from build123d import *

# Parameters (mm, degrees)
F1_DEPTH       = 15
F3_D           = 4.5
F3_CSINK_D     = 9
F3_CSINK_ANGLE = 90
F4_R           = 4
F5_R           = 1.5
F6_W           = 3
F6_H           = 8
F7_DEPTH       = 0.5
F8_R           = 1


with BuildPart() as f1:
    # F0 (on Right) → F1 (new body, symmetric)
    with BuildSketch(Plane.YZ):
        Polygon((0, 4.5), (0, 0), (9, 0), (9, 7.5), (-11, 7.5), (-11, 4.5), align=None)
    extrude(amount=F1_DEPTH, both=True)

    # F3 (through all)
    with Locations(Plane.XY.offset(7.5)):
        with Locations((-9, 3.5), (9, 3.5)):
            CounterSinkHole(F3_D / 2, F3_CSINK_D / 2, counter_sink_angle=F3_CSINK_ANGLE)

    # F4
    f4_edges = [f1.edges().sort_by_distance(p)[0] for p in [
        (15, -11, 6),
        (-15, -11, 6),
        (15, 0, 2.25),
        (-15, 0, 2.25),
        (-15, 9, 3.75),
        (15, 9, 3.75),
    ]]
    fillet(f4_edges, radius=F4_R)

    # F5
    f5_edges = [f1.edges().sort_by_distance(p)[0] for p in [
        (-15, -3.5, 4.5),
    ]]
    fillet(f5_edges, radius=F5_R)

    # F6 (on face) → F7 (cut)
    with BuildSketch(Plane.XY.offset(7.5)):
        with Locations((0, 3.5)):
            Rectangle(F6_W, F6_H)
    extrude(amount=-F7_DEPTH, mode=Mode.SUBTRACT)

    # F8
    f8_edges = [f1.edges().sort_by_distance(p)[0] for p in [
        (-1.5, 7.5, 7.25),
        (-1.5, -0.5, 7.25),
        (1.5, -0.5, 7.25),
        (1.5, 7.5, 7.25),
    ]]
    fillet(f8_edges, radius=F8_R)


solid = f1.part
Geometry: final body of the model. Coordinates: model frame, mm. A direction names the side the tool comes from. Coordinates: 2 decimals unless noted, no trailing zeros. Loops run counter-clockwise (first coordinate to the right, second up) from the corner with the lowest first, then second, coordinate; pieces in that order, holes last. Notation, with made-up numbers: (26, 68) - (82, 68) arc R19 ccw to (82, 77) - close; hole circle Ø1 at (26.5, -39). An arc over 180 degrees is marked (long way). One line per question, with ' | ' between items. Start each with the question number.
(1) Cut plane C-C on z = 2. Output: boundary loops of the cut face in (x, y).
(2) Draft query along X for faces 6 (the cylindrical face through (-0.15, -10.55, 4.93)), 7 (the cylindrical face through (14.55, -2.8, 4.93)), 8 (the flat face through (-15, 0.3, 6.3)), 9 (the cylindrical face through (10.786, 2.131, 2.588)). Return one class per face: +X half, -X half, draft (parallel to the pull), parting line (faces both ways), or undercut.
(3) Cut plane B-B on y = 3.5. Output: boundary loops of the cut face in (x, z).
(4) Reachability of faces 1 (the cylindrical face through (-13.797, 7.859, 3.802)), 2 (the cylindrical face through (-1.199, -0.215, 7.246)), 3 (the cylindrical face through (-14.55, -2.65, 4.93)), 4 (the cylindrical face through (13.797, 1.141, 2.291)), 5 (the cylindrical face through (13.797, 7.859, 3.802)) from +Z, -Z, +X, -X, +Y, -Y: full face, straight path, thin tool, end or side. Return the list, or none.
(5) First-contact query: pin 1 (1.5 mm diameter, centred on y = -8, z = 2, fed in from +X); pin 2 (1 mm diameter, centred on x = 5.5, z = 2, fed in from -Y); pin 3 (2 mm diameter, centred on x = 11.5, z = 2.5, fed in from +Y); pin 4 (8.5 mm diameter, centred on x = 4.5, y = -6, fed in from -Z). Flat tips, straight axial feed; report the tip coordinate or a pass-through.
(6) Cut plane D-D on y = -4.5. Output: boundary loops of the cut face in (x, z).
(7) Ray query, L1, parallel to X at y = 3.5, z = 2.15; L2, parallel to Y at x = -9, z = 1.4; L3, parallel to Z at x = -4.5, y = -7.25. Return the intervals inside material, ascending. Write a range as from..to.
(8) Cut plane A-A on x = -9. Output: boundary loops of the cut face in (y, z).
Here are the results:
1) outline: (-15, 4) arc R4 ccw to (-11, 0) - (11, 0) arc R4 ccw to (15, 4) - (15, 5) arc R4 ccw to (11, 9) - (-11, 9) arc R4 ccw to (-15, 5) - close; hole circle Ø4.5 at (-9, 3.5); hole circle Ø4.5 at (9, 3.5)
2) face 6: draft | face 7: +X half | face 8: -X half | face 9: undercut
3) outline: (-15, 6) arc R1.5 ccw to (-14.97, 5.69) - (-14.97, 0) - (-11.25, 0) - (-11.25, 5.25) - (-13.5, 7.5) - (-15, 7.5) - close; (-6.75, 0) - (6.75, 0) - (6.75, 5.25) - (4.5, 7.5) - (1.5, 7.5) - (1.5, 7) - (-1.5, 7) - (-1.5, 7.5) - (-4.5, 7.5) - (-6.75, 5.25) - close; (11.25, 0) - (14.97, 0) - (14.97, 5.69) arc R1.5 ccw to (15, 6) - (15, 7.5) - (13.5, 7.5) - (11.25, 5.25) - close
4) face 1: +Z, -Z, -X, +Y | face 2: +Z | face 3: -Z, -X, -Y | face 4: -Z, +X, -Y | face 5: +Z, -Z, +X, +Y
5) pin 1: through | pin 2: y = 0 | pin 3: y = 9 | pin 4: z = 4.5
6) outline: (-15, 6) arc R1.5 ccw to (-13.5, 4.5) - (13.5, 4.5) arc R1.5 ccw to (15, 6) - (15, 7.5) - (-15, 7.5) - close
7) L1: -14.97..-11.25, -6.75..6.75, 11.25..14.97 | L2: 0..1.25, 5.75..9 | L3: 4.5..7.5
8) outline: (-11, 6) arc R1.5 ccw to (-9.5, 4.5) - (0, 4.5) - (0, 0) - (1.25, 0) - (1.25, 5.25) - (-1, 7.5) - (-11, 7.5) - close; (5.75, 0) - (9, 0) - (9, 7.5) - (8, 7.5) - (5.75, 5.25) - close
